The figure shows three views and two pictorial views of one solid part (mm, origin at its lowest corner). Answer the questions. Coordinates: 2 decimals unless noted, no trailing zeros. Use CSV: the item, a comma, the result in double quotes.
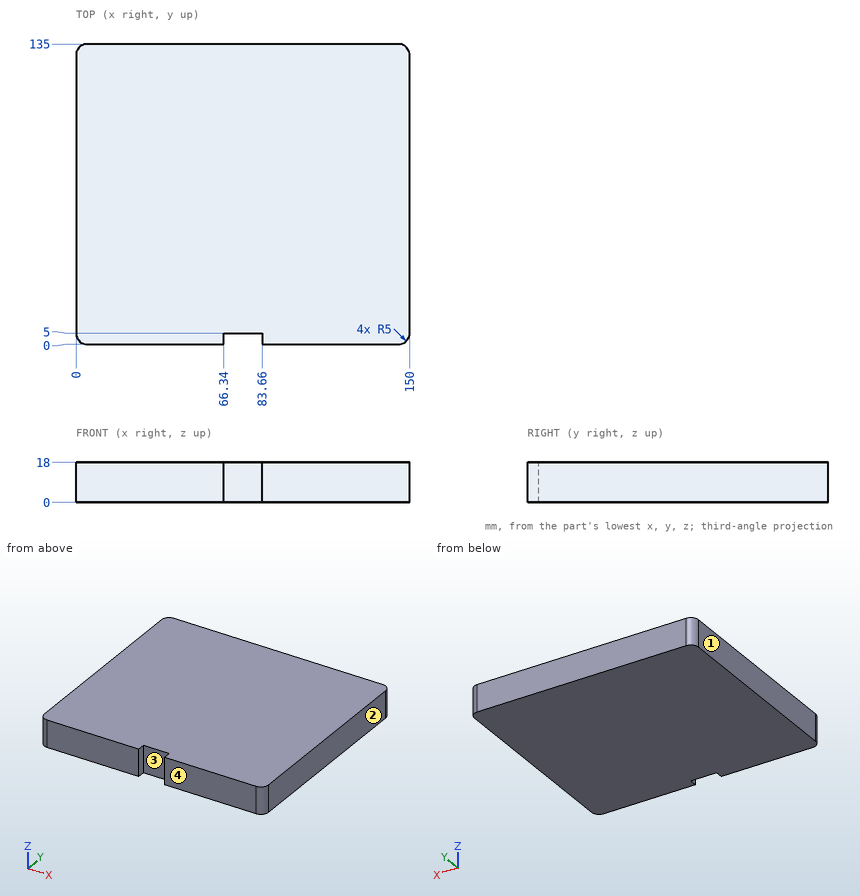
Item 1: Given pin 1 (5 mm diameter, centred on x = 47.5, y = 90.5, fed in from -Z), flat-ended and moving along its own axis, determine where the tip first touches the part or whether it passes through.
Answer:
pin 1,"stops at z = 0"
Item 2: For a pull along X with two mould halves and no side action, classify the marked faces 1, 2, 3 and 4 as released by +X, released by -X, zero draft, split by the parting line, or undercut.
Answer:
face 1,"released by -X"
face 2,"released by +X"
face 3,"undercut"
face 4,"zero draft"
Item 3: Consider probe 1 along Y at (x, z) = (68, 8). Determine where the line is inside the solid, lowest interval first.
Answer:
probe 1,"y = 5 to 135"
